```python
from build123d import *

# Parameters (mm, degrees)
SKETCH1_W                = 38.1
SKETCH1_H                = 266.7
BOSS_EXTRUDE1_DEPTH      = 7.9375
O_0_316_DIAMETER_HOLE1_D = 8.0264
SKETCH4_R                = 8.89
BOSS_EXTRUDE2_DEPTH      = 12.7


with BuildPart() as part:
    # Sketch1 → Boss-Extrude1 (new body)
    with BuildSketch(Plane.XY):
        Rectangle(SKETCH1_W, SKETCH1_H)
    extrude(amount=BOSS_EXTRUDE1_DEPTH)

    # O (0.316) Diameter Hole1 (through all)
    with Locations(Plane.XY.offset(7.9375)):
        with Locations((0, 114.3)):
            o_0_316_diameter_hole1 = Hole(O_0_316_DIAMETER_HOLE1_D / 2)

    # Mirror1: O (0.316) Diameter Hole1 across plane
    add(o_0_316_diameter_hole1.mirror(Plane.ZX), mode=Mode.SUBTRACT)

    # Sketch4 → Boss-Extrude2 (add)
    with BuildSketch(Plane.XY.offset(7.9375)):
        with Locations((-9.144, 95.25)):
            Circle(SKETCH4_R)
        with Locations((9.144, 95.25)):
            Circle(SKETCH4_R)
    extrude(amount=BOSS_EXTRUDE2_DEPTH)


solid = part.part
```
Can you work these out from the model? Positions are in its coordinate system, mm. A direction names the side the tool comes from. Round coordinates to 2 decimals unless told otherwise and drop trailing zeros. Loops run counter-clockwise (first coordinate to the right, second up) from the corner with the lowest first, then second, coordinate; pieces in that order, holes last. Notation, with made-up numbers: (-17, 41.25) -> (9, 41.25) arc R25 ccw to (9, 77.25) -> close; hole circle Ø5 at (52.25, -22.75). An arc over 180 degrees is marked (long way). One line per item, written item: value. Start each with the question number.
1. If we section it at B-B, the plane z = 12.75: Write out the boundary of the cut face in (x, y), then the cut area to 3 significant figures.
2. If we section it at C-C, the plane x = 10.5: Write out the boundary of the cut face in (y, z).
3. For pin 1 (6 mm diameter, centred on x = 7, y = 21.5, fed in from +Z); pin 2 (3 mm diameter, centred on x = -1, z = 10.5, fed in from -Y), each with a flat end and sliding along its axis, tell me the tip position at first contact or that it passes through.
4. For faces 5 (the cylindrical face through (13.92, 102.75, 14.2)), 6 (the flat face through (9, 95, 20.638)), which set-ups out of +Z, -Z, +X, -X, +Y, -Y let a thin tool reach every point of the face, with its end or its side?
5. If we mould it in two halves opening along X, with no side actions, what happens to faces 1 (the flat face through (-19.05, -2, 4)), 2 (the flat face through (0, 133.35, 4)), 3 (the cylindrical face through (-4.365, 102.746, 14.199)), 4 (the cylindrical face through (0.52, -118.28, 3.91))? For each: pulls with the +X half, pulls with the -X half, needs draft (parallel to the pull), parting line crosses it, or undercut.
6. If we section it at D-D, the plane y = -71.5: Write out the boundary of the cut face in (x, z).
7. If I drill on probe 1 along Y at (x, z) = (0, 3.25); probe 2 along Z at (x, y) = (-11, -43); probe 3 along Y at (x, z) = (15, 8.25), over which ranges is the centre line in solid material (lowest first)?
8. If we section it at A-A, the plane y = 114.3: Write out the boundary of the cut face in (x, z).
Calculated:
1. outline: circle Ø17.78 at (-9.14, 95.25); circle Ø17.78 at (9.14, 95.25)
1. area: 497 mm²
2. outline: (-133.35, 0) -> (133.35, 0) -> (133.35, 7.94) -> (104.04, 7.94) -> (104.04, 20.64) -> (86.46, 20.64) -> (86.46, 7.94) -> (-133.35, 7.94) -> close
3. pin 1: stops at z = 7.94
3. pin 2: stops at y = 89.34
4. face 5: +Z
4. face 6: +Z, +X, -X, +Y, -Y
5. face 1: pulls with the -X half
5. face 2: needs draft
5. face 3: undercut
5. face 4: undercut
6. outline: (-19.05, 0) -> (19.05, 0) -> (19.05, 7.94) -> (-19.05, 7.94) -> close
7. probe 1: y = -133.35 to -118.31, -110.29 to 110.29, 118.31 to 133.35
7. probe 2: z = 0 to 7.94
7. probe 3: y = 88.56 to 101.94
8. outline: (-19.05, 0) -> (-4.01, 0) -> (-4.01, 7.94) -> (-19.05, 7.94) -> close; (4.01, 0) -> (19.05, 0) -> (19.05, 7.94) -> (4.01, 7.94) -> close
